Autodesk Inventor part; units mm, degrees
ref_plane "XZ Plane" through (0, 0, 0) normal (0, 1, 0) x (-1, 0, 0)
ref_plane "XY Plane" through (0, 0, 0) normal (0, 0, 1) x (1, 0, 0)
sketch "Skizze1" plane through (0, 0, 0) normal (0, 0, 1) x (1, 0, 0)
  circle A0 centre (0, 0) radius 31
  circle A1 centre (0, 0) radius 29.5
  dimension "d0" = 62
  dimension "d1" = 59
extrude "Extrusion1" add sketch "Skizze1" along normal mid plane 300
sketch "Skizze2" plane through (0, 0, 0) normal (0, 1, 0) x (-1, 0, 0)
  line L0 (-10, 169.5773) -> (-10, -169.8146) construction
  line L1 (-74.8376, 0) -> (82.6362, 0) construction
  line L2 (-10, 75) -> (-10, -75)
  line L3 (-31, -150) -> (-31, 150)
  line L4 (31, 150) -> (-31, 150)
  line L5 (-31, -150) -> (31, -150)
  spline S0 degree 2 poles (-10, 75) (-18.1599, 136.3675) (-72.8449, 128.3193) knots 0 0 0 1 1 1
  spline S1 degree 2 poles (-10, -75) (-17.9565, -136.1553) (-74.8376, -130) knots 0 0 0 1 1 1
  line L6 (-72.8449, 128.3193) -> (-74.8376, -130)
  line L7 (-31, 120) -> (-31, 150)
  line L8 (-31, 150) -> (31, 150)
  line L9 (31, 150) -> (31, -150)
  line L10 (31, -150) -> (31, 150)
  line L11 (31, -150) -> (-31, -150)
  line L12 (-31, -150) -> (-31, -120)
  point P0 (0, 0)
  dimension "d4" = 10
  dimension "d5" = 150
  dimension "d6" = 30
  dimension "d7" = 30
extrude "Extrusion3" cut sketch "Skizze2" along normal mid plane 100 contours S0 L3 L4 L9 L5 S1 L2
ref_plane "Arbeitsebene1" through (26.5, 0, 0) normal (1, 0, 0) x (0, 1, 0)
properties part number "_3D-Druck"
Geometry check sheet. Reference: the model listing, model coordinates, mm. Coordinates: 2 decimals unless noted, no trailing zeros. Write each loop counter-clockwise with the first axis right and the second up, starting at its lowest first coordinate (ties: lowest second). Pieces come first, ordered by that corner, then holes. Notation, with made-up numbers: M -8.5,-12.5 L 9.5,-12.5 A8 ccw 9.5,-2.5 Z; hole C 89.25,9.25 d7. An arc over 180 degrees is marked long. Answer as a JSON object with one key per item and string values.
1. Go/stop test with flat-tipped pins: pin 1 Ø5 at (x, y) = (18.5, 21.5) entering from +Z; pin 2 Ø12 at (x, y) = (18, -2) entering from +Z; pin 3 Ø2 at (x, z) = (25, -54) entering from -Y; pin 4 Ø5 at (x, z) = (28, 42) entering from -Y. Record where each tip stops, or that it passes through.
Answers below:
{"pin 1": "stops at z = 108.82", "pin 2": "passes through", "pin 3": "stops at y = -19.62", "pin 4": "stops at y = -17.63"}
2. Section check A-A, the plane z = 70. Enter the section's corners in (x, y).
Answers below:
{"outline": "M 10,-29.34 A31 ccw 10,29.34 L 10,27.75 A29.5 cw 10,-27.75 Z"}
3. Scan lines: L1, parallel to Y at x = 14.75, z = 59; L2, parallel to Y at x = 13.5, z = -63; L3, parallel to X at y = -10, z = -57. Record each from-to range of solid material in increasing order.
Answers below:
{"L1": "y = -27.27 to -25.55, 25.55 to 27.27", "L2": "y = -27.91 to -26.23, 26.23 to 27.91", "L3": "x = 27.75 to 29.34"}
